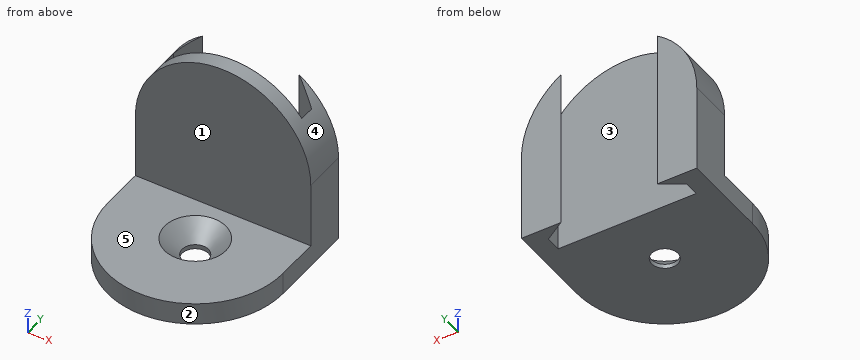
```python
from build123d import *

# Parameters (mm, degrees)
PAD_DEPTH    = 5
PAD001_DEPTH = 10
POCKET_DEPTH = 42
SKETCH003_R  = 3
HOLE_DEPTH   = 25
CHAMFER_SIZE = 4


with BuildPart() as part:
    # Sketch → Pad (new body)
    with BuildSketch(Plane.XY):
        with BuildLine():
            Line((-20, 0), (20, 0))
            Line((20, 0), (20, -20))
            ThreePointArc((-20, -20), (0, -40), (20, -20))
            Line((-20, 0), (-20, -20))
        make_face()
    extrude(amount=PAD_DEPTH)

    # Sketch001 (on Face1 of Pad) → Pad001 (join)
    with BuildSketch(Plane(origin=(0, 0, 0), x_dir=(-1, 0, 0), z_dir=(0, 1, 0))):
        with BuildLine():
            Line((-20, 20), (-20, 0))
            Line((-20, 0), (20, 0))
            Line((20, 0), (20, 20))
            ThreePointArc((20, 20), (0, 40), (-20, 20))
        make_face()
    extrude(amount=-PAD001_DEPTH)

    # Sketch002 (on Face4 of Pad001) → Pocket (cut)
    with BuildSketch(Plane(origin=(0, 0, 0), x_dir=(1, 0, 0), z_dir=(0, 0, -1))):
        Polygon((-15.75, 3), (-15.75, 6.5), (15.75, 6.5), (15.75, 3), (11, 0), (-11, 0), align=None)
    extrude(amount=-POCKET_DEPTH, mode=Mode.SUBTRACT)

    # Sketch003 → Hole (cut)
    with BuildSketch(Plane.XY.offset(5)):
        with Locations((0, -20)):
            Circle(SKETCH003_R)
    extrude(amount=-HOLE_DEPTH, mode=Mode.SUBTRACT)

    # Chamfer
    chamfer_edges = [part.edges().sort_by_distance(p)[0] for p in [
        (-3, -20, 5),
    ]]
    chamfer(chamfer_edges, length=CHAMFER_SIZE)


solid = part.part
```
Model file for the job. Use its own axes, mm. Face numbers are marked on the shaded views. A direction names the side the tool comes from. Coordinates: 2 decimals unless noted, no trailing zeros. Order: outer loops, then holes, each group sorted by start corner. A loop starts at its lowest first (then second) coordinate and runs counter-clockwise, first axis right, second up. Notation, with made-up numbers: (-20, 17) - (-16, 17) arc R24 ccw to (-16, 36) - close; hole circle Ø9 at (80, -30). An arc over 180 degrees is marked (long way). Return JSON: item names as keys, results as strings. Group by question number.
1) Saw through at C-C, the plane x = -17. Write the cut outline in (y, z).
2) Probe line 1 (Y direction, x = 0, z = 0.45); line 2 (X direction, y = -4.5, z = 18.5); line 3 (Y direction, x = 18.5, z = 25). List the from-to ranges inside material, lowest first. Write a range as from..to.
3) Tool access for the marked faces 4 and 5: list every direction of +Z, -Z, +X, -X, +Y, -Y with a clear straight run to the whole face (end or side of a thin tool).
4) Flat gauge pins, fed straight in: P1, Ø4, axis at y = -4, z = 22.5, coming from the -X side; P2, Ø1, axis at x = -12, y = -8.5, coming from the +Z side; P3, Ø1, axis at y = -10, z = 24.5, coming from the -X side; P4, Ø5, axis at x = 0, y = -20, coming from the +Z side. Where does each tip first touch, or does it go through?
5) Saw through at A-A, the plane x = 0. Write the cut outline in (y, z).
6) Saw through at D-D, the plane z = 27.5. Write the cut outline in (x, y).
7) Mould opens along X. For the marked faces 1, 2 and 3 say: released by +X, released by -X, zero draft, split by the parting line, or undercut.
8) Saw through at B-B, the plane z = 6. Write the cut outline in (x, y), plus the area to 4 significant figures.
Values found:
{
 "1": {"outline": "(-30.54, 0) - (0, 0) - (0, 30.54) - (-10, 30.54) - (-10, 5) - (-30.54, 5) - close"},
 "2": {"line 1": "y = -40..-23, -17..-6.5", "line 2": "x = -20..-15.75, 15.75..20", "line 3": "y = -10..0"},
 "3": {"face 4": "+Z, +Y, -Y", "face 5": "+Z, +X, -X, -Y"},
 "4": {"P1": "stops at x = -19.99", "P2": "stops at z = 36.36", "P3": "stops at x = -19.6", "P4": "passes through"},
 "5": {"outline": "(-40, 0) - (-23, 0) - (-23, 1) - (-27, 5) - (-40, 5) - close; (-17, 0) - (-6.5, 0) - (-6.5, 40) - (-10, 40) - (-10, 5) - (-13, 5) - (-17, 1) - close"},
 "6": {"outline": "(-18.54, -10) - (18.54, -10) - (18.54, 0) - (11, 0) - (15.75, -3) - (15.75, -6.5) - (-15.75, -6.5) - (-15.75, -3) - (-11, 0) - (-18.54, 0) - close"},
 "7": {"face 1": "zero draft", "face 2": "split by the parting line", "face 3": "undercut"},
 "8": {"outline": "(-20, -10) - (20, -10) - (20, 0) - (11, 0) - (15.75, -3) - (15.75, -6.5) - (-15.75, -6.5) - (-15.75, -3) - (-11, 0) - (-20, 0) - close", "area": "209.5 mm²"}
}
